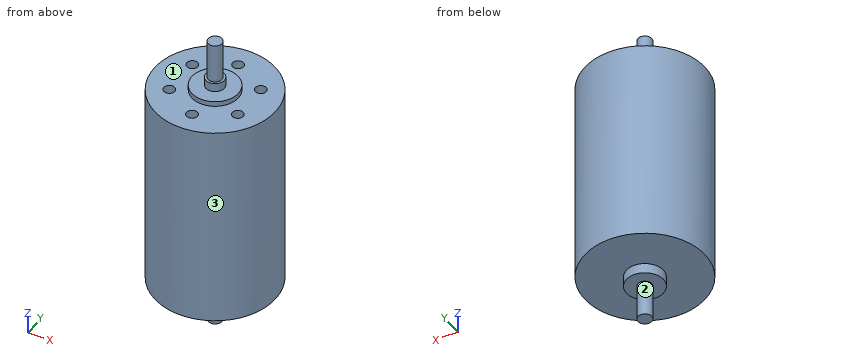
```python
from build123d import *

# Parameters (mm, degrees)
SKETCH1_R                        = 13
BOSS_EXTRUDE1_DEPTH              = 22.35
SKETCH2_R                        = 5
BOSS_EXTRUDE2_DEPTH              = 1.1
SKETCH3_R                        = 2
BOSS_EXTRUDE3_DEPTH              = 1.9
SKETCH4_R                        = 1.5
BOSS_EXTRUDE4_DEPTH              = 8.55
SKETCH5_R                        = 4
BOSS_EXTRUDE5_DEPTH              = 2.2
SKETCH6_R                        = 1.5
BOSS_EXTRUDE6_DEPTH              = 7.8
F_42_0_0935_DIAMETER_HOLE1_D     = 2.3749
F_42_0_0935_DIAMETER_HOLE1_DEPTH = 12.7
F_42_0_0935_DIAMETER_HOLE1_TIP   = 0.713491942


with BuildPart() as part:
    # Sketch1 → Boss-Extrude1 (new body, symmetric)
    with BuildSketch(Plane(origin=(0, 0, 0), x_dir=(0, 1, 0), z_dir=(0, 0, 1))):
        Circle(SKETCH1_R)
    extrude(amount=BOSS_EXTRUDE1_DEPTH, both=True)

    # Sketch2 → Boss-Extrude2 (add)
    with BuildSketch(Plane.XY.offset(22.35)):
        Circle(SKETCH2_R)
    extrude(amount=BOSS_EXTRUDE2_DEPTH)

    # Sketch3 → Boss-Extrude3 (add)
    with BuildSketch(Plane.XY.offset(23.45)):
        Circle(SKETCH3_R)
    extrude(amount=BOSS_EXTRUDE3_DEPTH)

    # Sketch4 → Boss-Extrude4 (add)
    with BuildSketch(Plane.XY.offset(25.35)):
        Circle(SKETCH4_R)
    extrude(amount=BOSS_EXTRUDE4_DEPTH)

    # Sketch5 → Boss-Extrude5 (add)
    with BuildSketch(Plane(origin=(0, 0, -22.35), x_dir=(1, 0, 0), z_dir=(0, 0, -1))):
        Circle(SKETCH5_R)
    extrude(amount=BOSS_EXTRUDE5_DEPTH)

    # Sketch6 → Boss-Extrude6 (add)
    with BuildSketch(Plane(origin=(0, 0, -24.55), x_dir=(1, 0, 0), z_dir=(0, 0, -1))):
        Circle(SKETCH6_R)
    extrude(amount=BOSS_EXTRUDE6_DEPTH)

    # #42 (0.0935) Diameter Hole1
    with Locations(Plane.XY.offset(22.35)):
        with Locations((7.361215932, -4.25), (0, 8.5), (-7.361215932, 4.25), (-7.361215932, -4.25), (7.361215932, 4.25), (0, -8.5)):
            Hole(F_42_0_0935_DIAMETER_HOLE1_D / 2, depth=F_42_0_0935_DIAMETER_HOLE1_DEPTH)
            with Locations((0, 0, -(F_42_0_0935_DIAMETER_HOLE1_DEPTH + F_42_0_0935_DIAMETER_HOLE1_TIP / 2))):  # 118° drill point
                Cone(0, F_42_0_0935_DIAMETER_HOLE1_D / 2, F_42_0_0935_DIAMETER_HOLE1_TIP, mode=Mode.SUBTRACT)


solid = part.part
```
Source: CAD feature listing. Evaluate the final solid. Frame: model axes, mm. Face numbers are marked on the shaded views. A direction names the side the tool comes from. Give positions to 0.01 mm unless a question says otherwise; leave off trailing zeros. Write each loop counter-clockwise with the first axis right and the second up, starting at its lowest first coordinate (ties: lowest second). Pieces come first, ordered by that corner, then holes.
1. Section query C-C (x = 10). Return the cut outline in (y, z).
2. Section query B-B (z = -11). Return the cut outline in (x, y).
3. Section query D-D (x = -9.75). Return the cut outline in (y, z).
4. Section query A-A (y = 0). Return the cut outline in (x, z), then the cut area to 3 significant figures.
5. Material intervals for line 1 along X through (y, z) = (4.25, 13); line 2 along Y through (x, z) = (0, 16.5); line 3 along Y through (x, z) = (-8, 17), sorted ascending.
6. First-contact query: pin 1 (4 mm diameter, centred on x = 7.36, y = -4.25, fed in from +Z); pin 2 (1.5 mm diameter, centred on x = 0.5, y = -9.5, fed in from -Z); pin 3 (2 mm diameter, centred on x = 7.36, y = 4.25, fed in from +Z). Flat tips, straight axial feed; report the tip coordinate or a pass-through.
7. Access query for the marked faces 1, 2 and 3. Directions: +Z, -Z, +X, -X, +Y, -Y. A direction counts if a zero-diameter tool reaches every point of the face in a straight line with its end or side. Return the directions, or none.
Output values:
1. outline: (-8.31, -22.35) - (8.31, -22.35) - (8.31, 22.35) - (-8.31, 22.35) - close
2. outline: circle Ø26 at (0, 0)
3. outline: (-8.6, -22.35) - (8.6, -22.35) - (8.6, 22.35) - (-8.6, 22.35) - close
4. outline: (-13, -22.35) - (-4, -22.35) - (-4, -24.55) - (-1.5, -24.55) - (-1.5, -32.35) - (1.5, -32.35) - (1.5, -24.55) - (4, -24.55) - (4, -22.35) - (13, -22.35) - (13, 22.35) - (5, 22.35) - (5, 23.45) - (2, 23.45) - (2, 25.35) - (1.5, 25.35) - (1.5, 33.9) - (-1.5, 33.9) - (-1.5, 25.35) - (-2, 25.35) - (-2, 23.45) - (-5, 23.45) - (-5, 22.35) - (-13, 22.35) - close
4. area: 1,250 mm2
5. line 1: x = -12.29 to -8.55, -6.17 to 6.17, 8.55 to 12.29
5. line 2: y = -13 to -9.69, -7.31 to 7.31, 9.69 to 13
5. line 3: y = -10.25 to -5.25, -3.25 to 3.25, 5.25 to 10.25
6. pin 1: stops at z = 22.35
6. pin 2: stops at z = -22.35
6. pin 3: stops at z = 9.54
7. face 1: +Z
7. face 2: -Z
7. face 3: +Z, -Z
